Could you check a few things on this model? Use its own coordinates, in mm. A direction names the side the tool comes from. Give positions to 0.01 mm unless a question says otherwise; leave off trailing zeros. Order: outer loops, then holes, each group sorted by start corner. A loop starts at its lowest first (then second) coordinate and runs counter-clockwise, first axis right, second up.
from build123d import *

# Parameters (mm, degrees)
PAD003_DEPTH    = 7
POCKET002_DEPTH = 7
POCKET008_DEPTH = 10
POCKET009_DEPTH = 6
SKETCH020_W     = 66
SKETCH020_H     = 2.5
SKETCH020_W_2   = 2.5
SKETCH020_H_2   = 38
PAD009_DEPTH    = 1
SKETCH021_W     = 2
SKETCH021_H     = 4
PAD010_DEPTH    = 1
CHAMFER_SIZE    = 0.45
FILLET001_R     = 1
SKETCH022_W     = 75.000016
SKETCH022_H     = 2
POCKET010_DEPTH = 1


with BuildPart() as part:
    # Sketch006 → Pad003 (new body)
    with BuildSketch(Plane.XY):
        with BuildLine():
            Line((-35, -37.5), (34.999998, -37.5))
            ThreePointArc((34.999998, -37.5), (36.767767, -36.767767), (37.5, -34.999999))
            Line((37.5, 35.000016), (37.5, -34.999999))
            ThreePointArc((37.5, 35.000016), (36.767767, 36.767767), (35.000016, 37.5))
            Line((35.000016, 37.5), (-35, 37.5))
            ThreePointArc((-35, 37.5), (-36.767767, 36.767767), (-37.5, 34.999999))
            Line((-37.5, 34.999999), (-37.5, -35))
            ThreePointArc((-37.5, -35), (-36.767767, -36.767767), (-35, -37.5))
        make_face()
    extrude(amount=PAD003_DEPTH)

    # Sketch007 → Pocket002 (cut)
    with BuildSketch(Plane(origin=(0, 0, 0), x_dir=(1, 0, 0), z_dir=(0, 0, -1))):
        with BuildLine():
            Line((-15, 20), (15, 20))
            ThreePointArc((15, -20), (25, 0), (15, 20))
            Line((-15, -20), (15, -20))
            ThreePointArc((-15, 20), (-25, 0), (-15, -20))
        make_face()
    extrude(amount=-POCKET002_DEPTH, mode=Mode.SUBTRACT)

    # Sketch009 → Pocket008 (cut)
    with BuildSketch(Plane(origin=(0, 0, 0), x_dir=(1, 0, 0), z_dir=(0, 0, -1))):
        with BuildLine():
            ThreePointArc((-27.96854, 4.931608), (-28.4, 0), (-27.96854, -4.931608))
            ThreePointArc((-31.119925, -5.487282), (-29.266396, -6.785138), (-27.96854, -4.931608))
            ThreePointArc((-31.119925, 5.487282), (-31.6, 0), (-31.119925, -5.487282))
            ThreePointArc((-27.96854, 4.931608), (-29.266396, 6.785138), (-31.119925, 5.487282))
        make_face()
        with BuildLine():
            ThreePointArc((27.96854, -4.931608), (28.4, -4e-06), (27.968542, 4.9316))
            ThreePointArc((31.119923, 5.487291), (29.266387, 6.785136), (27.968542, 4.9316))
            ThreePointArc((31.119925, -5.487282), (31.6, 5e-06), (31.119923, 5.487291))
            ThreePointArc((27.96854, -4.931608), (29.266396, -6.785138), (31.119925, -5.487282))
        make_face()
    extrude(amount=-POCKET008_DEPTH, mode=Mode.SUBTRACT)

    # Sketch019 → Pocket009 (cut)
    with BuildSketch(Plane.XY.offset(7)):
        Polygon((35, -35), (33, -35), (33, -37.5), (-33, -37.5), (-33, -35), (-35, -35), (-35, -33), (-37.5, -33), (-37.5, 5), (-35, 5), (-35, 35), (-33, 35), (-33, 37.5), (33, 37.5), (33, 35), (35, 35), (35, 5), (37.5, 5), (37.5, -33), (35, -33), align=None)
    extrude(amount=-POCKET009_DEPTH, mode=Mode.SUBTRACT)

    # Sketch020 → Pad009 (new body)
    with BuildSketch(Plane.XY.offset(1)):
        with Locations((0, -36.25)):
            Rectangle(SKETCH020_W, SKETCH020_H)
        with Locations((36.25, -14)):
            Rectangle(SKETCH020_W_2, SKETCH020_H_2)
        with Locations((0, 36.25)):
            Rectangle(SKETCH020_W, SKETCH020_H)
        with Locations((-36.25, -14)):
            Rectangle(SKETCH020_W_2, SKETCH020_H_2)
    extrude(amount=PAD009_DEPTH)

    # Sketch021 → Pad010 (new body)
    with BuildSketch(Plane.XZ.offset(37.5)):
        with Locations((-34, 3)):
            Rectangle(SKETCH021_W, SKETCH021_H)
        with Locations((34, 3)):
            Rectangle(SKETCH021_W, SKETCH021_H)
    extrude(amount=PAD010_DEPTH)

    # Chamfer
    chamfer_edges = [part.edges().sort_by_distance(p)[0] for p in [
        (-34, -38.5, 5),
        (-34, -38.5, 1),
        (34, -38.5, 5),
        (34, -38.5, 1),
    ]]
    chamfer(chamfer_edges, length=CHAMFER_SIZE)

    # Fillet001
    fillet001_edges = [part.edges().sort_by_distance(p)[0] for p in [
        (-37.5, -34, 7),
        (-36.767767, -36.767767, 7),
        (-34, -37.5, 7),
        (33.999999, -37.5, 7),
        (36.767767, -36.767767, 7),
        (37.5, -34, 7),
        (-37.5, 20, 7),
        (-36.767767, 36.767767, 7),
        (-34, 37.5, 7),
        (34.000008, 37.5, 7),
        (36.767767, 36.767767, 7),
        (37.5, 20.000008, 7),
    ]]
    fillet(fillet001_edges, radius=FILLET001_R)

    # Sketch022 → Pocket010 (cut)
    with BuildSketch(Plane(origin=(0, 37.5, 0), x_dir=(-1, 0, 0), z_dir=(0, 1, 0))):
        with Locations((-8e-06, 3)):
            Rectangle(SKETCH022_W, SKETCH022_H)
    extrude(amount=-POCKET010_DEPTH, mode=Mode.SUBTRACT)


solid = part.part
Item 1: For faces 4 (the flat face through (36, -33, 5)), 5 (the cylindrical face through (29.23, 6.78, 0.49)), 6 (the flat face through (-35, 15, 4)), which set-ups out of +Z, -Z, +X, -X, +Y, -Y let a thin tool reach every point of the face, with its end or its side?
Findings:
face 4: +Z, +X, -X
face 5: +Z, -Z
face 6: +Z
Item 2: Imagine slicing it at B-B on x = -9.5. List the corners of the cut face in (y, z) for me, then the cut area to 3 significant figures.
Findings:
outline: (-37.5, 0) - (-20, 0) - (-20, 1) - (-35, 1) - (-35, 2) - (-37.5, 2) - close; (20, 0) - (37.5, 0) - (37.5, 2) - (35, 2) - (35, 1) - (20, 1) - close
area: 40.0 mm2
Item 3: Imagine slicing it at D-D on y = 32. List the corners of the cut face in (x, z) for me.
Findings:
outline: (-37.5, 0) - (37.5, 0) - (37.5, 6) arc R1 ccw to (36.5, 7) - (35, 7) - (35, 1) - (-35, 1) - (-35, 7) - (-36.5, 7) arc R1 ccw to (-37.5, 6) - close
Item 4: We'd pull the mould along Y, two halves only. Please class faces 1 (the flat face through (-33, -37, 4)), 2 (the flat face through (36, -14, 2)), 3 (the cylindrical face through (37.28, 36.03, 2.96)): +Y half, -Y half, draft (parallel to the pull), parting line (faces both ways), or undercut.
Findings:
face 1: draft
face 2: undercut
face 3: +Y half
Item 5: For pin 1 (3 mm diameter, centred on x = -36.5, y = -20, fed in from +Z); pin 2 (0.8 mm diameter, centred on y = -38, z = 4, fed in from +X); pin 3 (0.8 mm diameter, centred on x = 35.5, z = 4.5, fed in from -Y); pin 4 (2 mm diameter, centred on x = 15, y = -26.5, fed in from -Z), each with a flat end and sliding along its axis, tell me the tip position at first contact or that it passes through.
Findings:
pin 1: stops at z = 2
pin 2: stops at x = 35
pin 3: stops at y = -37.5
pin 4: stops at z = 0
Item 6: Imagine slicing it at A-A on z = 3. Give the number of separate pieces and of enclosed holes in the cut face, then the cut area to 3 significant figures.
Findings:
separate pieces: 4
enclosed holes: 0
area: 197 mm2
Item 7: Please list where these lines run through material, in increasing order: line 1 along Y through (x, z) = (31.5, 1.5); line 2 along Z through (x, y) = (2.5, 28).
Findings:
line 1: y = -37.5 to -35, 35 to 37.5
line 2: z = 0 to 1
Item 8: Imagine slicing it at C-C on y = -11. List the corners of the cut face in (x, z) for me, then the cut area to 3 significant figures.
Findings:
outline: (-37.5, 0) - (-22.45, 0) - (-22.45, 1) - (-35, 1) - (-35, 2) - (-37.5, 2) - close; (22.45, 0) - (37.5, 0) - (37.5, 2) - (35, 2) - (35, 1) - (22.45, 1) - close
area: 35.1 mm2
